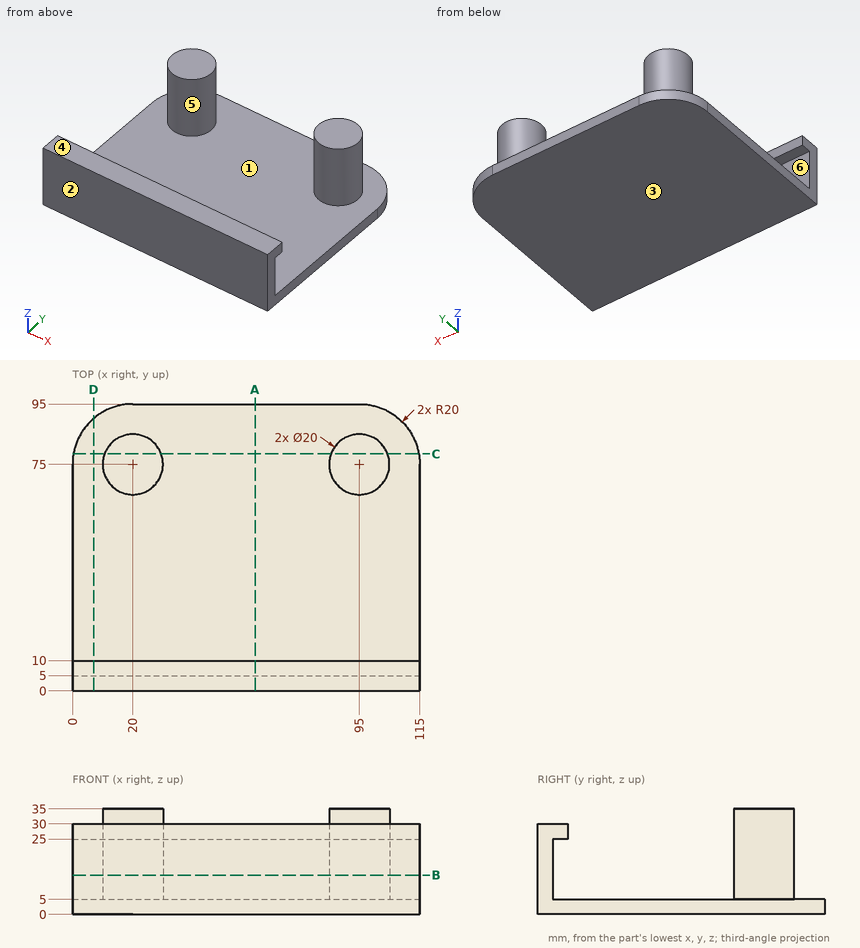
Part print with two shaded views. Sizes in mm from the minimum x, y, z corner. A direction names the side the tool comes from. Round coordinates to 2 decimals unless told otherwise and drop trailing zeros. Loops run counter-clockwise (first coordinate to the right, second up) from the corner with the lowest first, then second, coordinate; pieces in that order, holes last. Notation, with made-up numbers: (2, 39) - (23, 39) arc R19 cw to (23, 73) - close; hole circle Ø8 at (-36, 17.25). An arc over 180 degrees is marked (long way). Put each result on its own line as item: value.
1. Slice it at C-C on y = 78.5. List the corners of the cut face in (x, z).
Geometry check:
outline: (0.31, 0) - (114.69, 0) - (114.69, 5) - (104.37, 5) - (104.37, 35) - (85.63, 35) - (85.63, 5) - (29.37, 5) - (29.37, 35) - (10.63, 35) - (10.63, 5) - (0.31, 5) - close
2. Two-plate mould, pull along Y, no slides. Class the marked faces 1, 2 and 3: released by +Y, released by -Y, zero draft, split by the parting line, or undercut.
Geometry check:
face 1: undercut
face 2: released by -Y
face 3: zero draft
3. Pin check, flat tips, straight feed: P1, Ø8, axis at x = 72.5, y = 6.5, coming from the +Z side; P2, Ø8, axis at y = 70.5, z = 29.5, coming from the +X side; P3, Ø8, axis at y = 81.5, z = 13.5, coming from the +X side. Stop position of each tip, or through.
Geometry check:
P1: z = 30
P2: x = 104.99
P3: x = 104.68
4. 3-axis set-ups, long thin cutter, end or side, ignore diameter. For the marked faces 4, 5 and 6: which of +Z, -Z, +X, -X, +Y, -Y reach the whole face in a straight line?
Geometry check:
face 4: +Z, +X, -X, -Y
face 5: +Z
face 6: +X, -X
5. Slice it at D-D on x = 7. List the corners of the cut face in (y, z).
Geometry check:
outline: (0, 0) - (90.2, 0) - (90.2, 5) - (5, 5) - (5, 25) - (10, 25) - (10, 30) - (0, 30) - close
6. Wall check: line 1 (Z direction, x = 85, y = 68); line 2 (Z direction, x = 17, y = 7). Give the ranges that are in metal, low to high.
Geometry check:
line 1: 0 to 5
line 2: 0 to 5, 25 to 30
7. Slice it at A-A on x = 60.5. List the corners of the cut face in (y, z), and give its area (3 significant figures).
Geometry check:
outline: (0, 0) - (95, 0) - (95, 5) - (5, 5) - (5, 25) - (10, 25) - (10, 30) - (0, 30) - close
area: 625 mm²
8. Slice it at B-B on z = 13. List the corners of the cut face in (x, y), and give its area (3 significant figures).
Geometry check:
outline: (0, 0) - (115, 0) - (115, 5) - (0, 5) - close; circle Ø20 at (20, 75); circle Ø20 at (95, 75)
area: 1,200 mm²
